Verification items for the finished model (mm, model axes). A direction names the side the tool comes from. Coordinates: 2 decimals unless noted, no trailing zeros. Loops run counter-clockwise (first coordinate to the right, second up) from the corner with the lowest first, then second, coordinate; pieces in that order, holes last. Notation, with made-up numbers: (60.5, 22.25) -> (94.5, 22.25) arc R12 cw to (94.5, 40.25) -> close; hole circle Ø7 at (-3, -12). An arc over 180 degrees is marked (long way). Answer as a JSON object with one key per item and string values. Group by question number.
Q1. Cross-section at A-A on y = -78. Record the boundary of the cut face in (x, z).
Q2. Scan lines: L1, parallel to Z at x = 1.05, y = -129; L2, parallel to Y at x = 0.35, z = -9; L3, parallel to Z at x = 1.95, y = 26.5. Record each from-to range of solid material in increasing order.
Q3. Release check for a two-part mould opening along Z. For faces 4 (the flat face through (3, -21.727, 1)), 5 (the flat face through (3, -142, -21.812)), 6 (the flat face through (5.13, -50, -50)) record: released by +Z, released by -Z, zero draft, split by the parting line, or undercut.
Q4. Cross-section at B-B on z = -101.5. Record the boundary of the cut face in (x, y), and give its area (3 significant figures).
Q5. Cross-section at C-C on x = 2.1. Give the number of separate pieces and of enclosed holes in the cut face, and give its area (3 significant figures).
Q6. Set-up check for faces 1 (the flat face through (3, -138, -109.192)), 2 (the flat face through (3, -12.372, 1)), 3 (the flat face through (3, 36, -112.189)): record each of +Z, -Z, +X, -X, +Y, -Y from which the full face is reachable in a straight line by a thin tool's end or side.
Q7. Gauge pin test, flat ends, axial feed: pin 1 Ø1.5 at (x, z) = (2.5, -8.5) entering from -Y; pin 2 Ø4.5 at (y, z) = (-114.09, 27.44) entering from +X; pin 3 Ø1 at (x, z) = (1, -0.5) entering from +Y; pin 4 Ø2.5 at (x, z) = (2, 8) entering from -Y. Record the tip position at first contact, or that the pin passes through.
```python
from build123d import *

# Parameters (mm, degrees)
SKETCH1_W                  = 173.89
SKETCH1_H                  = 177.8
BOSS_EXTRUDE1_DEPTH        = 5.13
SKETCH6_W                  = 5.13
SKETCH6_H                  = 58.88
TEETH_DEPTH                = 5.13
T_SLOT_DEPTH               = 5.13
T_SLOT_PATTERN_COUNT       = 2
T_SLOT_PATTERN_PITCH       = 118.88
T_SLOT_BOTTOM_COPY_1_DEPTH = 5.13
SKETCH3_W                  = 26.322180797
SKETCH3_H                  = 49.826019937
POWER_PORT_DEPTH           = 5.13
SKETCH7_R                  = 1.7145
POWER_SUPPLY_SCREWS_DEPTH  = 5.13
SKETCH4_W                  = 41
SKETCH4_H                  = 9.354563129
FAN_VENT_DEPTH             = 5.13
LPATTERN3_COUNT            = 4
LPATTERN3_PITCH            = 12
SKETCH5_W                  = 13.315736025
SKETCH5_H                  = 12.842697729
USB_PORT_DEPTH             = 5.13
SKETCH11_W                 = 5.13
SKETCH11_H                 = 58.88
BOSS_EXTRUDE2_DEPTH        = 5.13
LPATTERN4_COUNT            = 2
LPATTERN4_PITCH            = 51
LPATTERN4_COUNT_DIR2       = 2
LPATTERN4_PITCH_DIR2       = 113.5


with BuildPart() as part:
    # Sketch1 → Boss-Extrude1 (new body)
    with BuildSketch(Plane(origin=(0, 0, 0), x_dir=(0, 0, -1), z_dir=(1, 0, 0))):
        with Locations((51.252197546, -50.943101868)):
            Rectangle(SKETCH1_W, SKETCH1_H)
    extrude(amount=BOSS_EXTRUDE1_DEPTH)

    # Sketch6 → teeth (add)
    with BuildSketch(Plane(origin=(0, 37.956898132, 0), x_dir=(1, 0, 0), z_dir=(0, 1, 0))):
        with Locations((2.565, 51.252197546)):
            Rectangle(SKETCH6_W, SKETCH6_H)
    extrude(amount=TEETH_DEPTH)

    # Sketch2 → t-slot (cut)
    with BuildSketch(Plane(origin=(5.13, 0, 0), x_dir=(0, 0, -1), z_dir=(1, 0, 0))):
        Polygon((-9.687802454, 37.956898132), (-6.690802454, 37.956898132), (-6.690802454, 33.961898132), (-5.331802454, 33.961898132), (-5.331802454, 31.794898132), (-6.690802454, 31.794898132), (-6.690802454, 25.587898132), (-9.687802454, 25.587898132), (-9.687802454, 31.794898132), (-11.046802454, 31.794898132), (-11.046802454, 33.961898132), (-9.687802454, 33.961898132), align=None)
    t_slot = extrude(amount=-T_SLOT_DEPTH, mode=Mode.SUBTRACT)

    # t-slot pattern: t-slot ×2
    with Locations(*[(0, 0, -i * T_SLOT_PATTERN_PITCH) for i in range(1, T_SLOT_PATTERN_COUNT)]):
        add(t_slot, mode=Mode.SUBTRACT)

    # t-slot bottom: t-slot across plane
    add(t_slot.mirror(Plane(origin=(0, -50.943101868, 0), x_dir=(0, 0, 1), z_dir=(0, -1, 0))), mode=Mode.SUBTRACT)

    # t-slot bottom copy 1 sketch → t-slot bottom copy 1 (cut)
    with BuildSketch(Plane(origin=(5.13, -101.886203737, -118.88), x_dir=(0, 0, -1), z_dir=(1, 0, 0))):
        Polygon((-9.687802454, -37.956898132), (-6.690802454, -37.956898132), (-6.690802454, -33.961898132), (-5.331802454, -33.961898132), (-5.331802454, -31.794898132), (-6.690802454, -31.794898132), (-6.690802454, -25.587898132), (-9.687802454, -25.587898132), (-9.687802454, -31.794898132), (-11.046802454, -31.794898132), (-11.046802454, -33.961898132), (-9.687802454, -33.961898132), align=None)
    extrude(amount=-T_SLOT_BOTTOM_COPY_1_DEPTH, mode=Mode.SUBTRACT)

    # Sketch3 → power port (cut)
    with BuildSketch(Plane(origin=(5.13, 0, 0), x_dir=(0, 0, -1), z_dir=(1, 0, 0))):
        with Locations((-7.323344752, -75.302440375)):
            Rectangle(SKETCH3_W, SKETCH3_H)
    extrude(amount=-POWER_PORT_DEPTH, mode=Mode.SUBTRACT)

    # Sketch7 → Power supply screws (cut)
    with BuildSketch(Plane(origin=(5.13, 0, 0), x_dir=(0, 0, -1), z_dir=(1, 0, 0))):
        with Locations((-27.442802454, -0.593101868)):
            Circle(SKETCH7_R)
    power_supply_screws = extrude(amount=-POWER_SUPPLY_SCREWS_DEPTH, mode=Mode.SUBTRACT)

    # Sketch4 → fan vent (cut)
    with BuildSketch(Plane(origin=(5.13, 0, 0), x_dir=(0, 0, -1), z_dir=(1, 0, 0))):
        with Locations((-0.321795885, -5.04966493)):
            Rectangle(SKETCH4_W, SKETCH4_H)
    fan_vent = extrude(amount=-FAN_VENT_DEPTH, mode=Mode.SUBTRACT)

    # LPattern3: fan vent ×4
    with Locations(*[(0, -i * LPATTERN3_PITCH, 0) for i in range(1, LPATTERN3_COUNT)]):
        add(fan_vent, mode=Mode.SUBTRACT)

    # Sketch5 → USB port (cut)
    with BuildSketch(Plane(origin=(5.13, 0, 0), x_dir=(0, 0, -1), z_dir=(1, 0, 0))):
        with Locations((90.737265655, -129.344754623)):
            Rectangle(SKETCH5_W, SKETCH5_H)
    extrude(amount=-USB_PORT_DEPTH, mode=Mode.SUBTRACT)

    # Sketch11 → Boss-Extrude2 (add)
    with BuildSketch(Plane.XZ.offset(139.843101868)):
        with Locations((2.565, -51.252197546)):
            Rectangle(SKETCH11_W, SKETCH11_H)
    extrude(amount=BOSS_EXTRUDE2_DEPTH)

    # LPattern4: Power supply screws 2 × 2
    with Locations(*[(0, -j * LPATTERN4_PITCH_DIR2, -i * LPATTERN4_PITCH) for i in range(LPATTERN4_COUNT) for j in range(LPATTERN4_COUNT_DIR2) if (i, j) != (0, 0)]):
        add(power_supply_screws, mode=Mode.SUBTRACT)


solid = part.part
```
Computed values:
{
 "1": {"outline": "(0, -138.2) -> (5.13, -138.2) -> (5.13, -5.84) -> (0, -5.84) -> close; (0, 20.48) -> (5.13, 20.48) -> (5.13, 35.69) -> (0, 35.69) -> close"},
 "2": {"L1": "z = -138.2 to -112.19, -109.19 to -97.4, -84.08 to 6.69, 9.69 to 35.69", "L2": "y = -139.84 to -45.73, -36.37 to -33.73, -24.37 to -21.73, -12.37 to -9.73, -0.37 to 37.96", "L3": "z = -138.2 to -112.19, -109.19 to 6.69, 9.69 to 35.69"},
 "3": {"face 4": "undercut", "face 5": "released by +Z", "face 6": "zero draft"},
 "4": {"outline": "(0, -139.84) -> (5.13, -139.84) -> (5.13, 37.96) -> (0, 37.96) -> close", "area": "912 mm²"},
 "5": {"separate pieces": "1", "enclosed holes": "10", "area": "28,300 mm²"},
 "6": {"face 1": "+X, -X, -Y", "face 2": "+X, -X", "face 3": "+X, -X, +Y"},
 "7": {"pin 1": "stops at y = -139.84", "pin 2": "stops at x = 5.13", "pin 3": "stops at y = 37.96", "pin 4": "stops at y = -127.47"}
}
